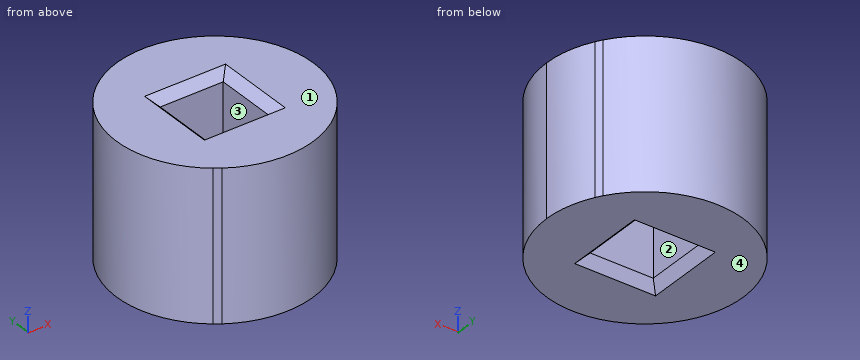
```python
from build123d import *

# Parameters (mm, degrees)
F0_W     = 4.23
F0_H     = 4.23
F1_DEPTH = 10
F2_SIZE  = 0.6


# Not quite as in the source:
# - two fillets or chamfers of one size are made in one step


with BuildPart() as f1:
    # F0 (on Top) → F1 (new body)
    with BuildSketch(Plane.XY):
        with BuildLine():
            Line((-18.6, 10.6), (-9.2461221228, 10.6))
            ThreePointArc((-9.2461221228, 10.6), (-9.3644866857, 10.802164009), (-9.4899513299, 11))
            Line((-9.4899513299, 11), (-19, 11))
            Line((-19, 11), (-19, 2.1171452511))
            ThreePointArc((-19, 2.1171452511), (-18.8026143682, 1.9724540765), (-18.6, 1.8351804761))
            Line((-18.6, 1.8351804761), (-18.6, 10.6))
        make_face()
        with BuildLine():
            Line((-19, 11), (-9.4899513299, 11))
            ThreePointArc((-9.4899513299, 11), (-19.5051458211, 12.1901489162), (-19, 2.1171452511))
            Line((-19, 2.1171452511), (-19, 11))
        make_face()
        with BuildLine():
            ThreePointArc((-18.6, 1.8351804761), (-11.8535734555, 1.5651832687), (-8.4, 7.3669071504))
            ThreePointArc((-8.4, 7.3669071504), (-8.6150335165, 9.0378957815), (-9.2461221228, 10.6))
            Line((-9.2461221228, 10.6), (-18.6, 10.6))
            Line((-18.6, 10.6), (-18.6, 1.8351804761))
        make_face()
        with Locations((-15, 7.3669071504)):
            Rectangle(F0_W, F0_H, mode=Mode.SUBTRACT)
    extrude(amount=F1_DEPTH)

    # F2
    f2_edges = [f1.edges().sort_by_distance(p)[0] for p in [
        (-17.115, 7.366907, 10),
        (-15, 5.251907, 10),
        (-12.885, 7.366907, 10),
        (-15, 9.481907, 10),
        (-17.115, 7.366907, 0),
        (-15, 9.481907, 0),
        (-12.885, 7.366907, 0),
        (-15, 5.251907, 0),
    ]]
    chamfer(f2_edges, length=F2_SIZE)


solid = f1.part
```
Source: CAD feature listing. Evaluate the final solid. Frame: model axes, mm. Face numbers are marked on the shaded views. A direction names the side the tool comes from. Coordinates: 2 decimals unless noted, no trailing zeros. Loops run counter-clockwise (first coordinate to the right, second up) from the corner with the lowest first, then second, coordinate; pieces in that order, holes last. Notation, with made-up numbers: M -40,-22 L 4,-22 A31 ccw 4,15 Z; hole C -19.75,18.5 d3. An arc over 180 degrees is marked long. Use a Markdown table: item, result. Add a question column.
Q1. Section query C-C, the plane y = 11.5. Return loops of the section in (x, z), and give its area (3 significant figures).
Q2. Section query B-B, the plane x = -15. Return loops of the section in (y, z).
Q3. Access query for the marked faces 1 and 2. Directions: +Z, -Z, +X, -X, +Y, -Y. A direction counts if a zero-diameter tool reaches every point of the face in a straight line with its end or side. Return the directions, or none.
Q4. Section query D-D, the plane x = -10. Return loops of the section in (y, z), and give its area (3 significant figures).
Q5. Draft query along Y for the marked faces 3 and 4. Return one class per face: pulls with the +Y half, pulls with the -Y half, needs draft (parallel to the pull), parting line crosses it, or undercut.
Q6. First-contact query: pin 1 (6 mm diameter, centred on y = 11.5, z = 4, fed in from -X). Flat tip, straight axial feed; report the tip coordinate or a pass-through.
Q7. Material intervals for L1, parallel to Y at x = -15.25, z = 1; L2, parallel to Y at x = -14.5, z = 6.75; L3, parallel to X at y = 6.75, z = 5 (3 decimals), sorted ascending.
Q8. Section query A-A, the plane z = 9. Return loops of the section in (x, y) (3 decimals).
Result:
| question | item | result |
|---|---|---|
| 1 | outline | M -20.15,0 L -9.85,0 L -9.85,10 L -20.15,10 Z |
| 1 | area | 103 mm2 |
| 2 | outline | M 0.77,0 L 4.65,0 L 5.25,0.6 L 5.25,9.4 L 4.65,10 L 0.77,10 Z; M 9.48,0.6 L 10.08,0 L 13.97,0 L 13.97,10 L 10.08,10 L 9.48,9.4 Z |
| 3 | face 1 | +Z, +X, -X, +Y, -Y |
| 3 | face 2 | +Z, -Z |
| 4 | outline | M 3.06,0 L 11.68,0 L 11.68,10 L 3.06,10 Z |
| 4 | area | 86.2 mm2 |
| 5 | face 3 | undercut |
| 5 | face 4 | needs draft |
| 6 | pin 1 | stops at x = -21.5 |
| 7 | L1 | y = 0.77 to 5.25, 9.48 to 13.96 |
| 7 | L2 | y = 0.79 to 5.25, 9.48 to 13.95 |
| 7 | L3 | x = -21.571 to -17.115, -12.885 to -8.429 |
| 8 | outline | C -15,7.367 d13.2; hole M -17.115,5.252 L -12.885,5.252 L -12.885,9.482 L -17.115,9.482 Z |
